Design review of the part shown in the three views and the two pictorial views. Dimensions are in mm from the part's minimum x, y and z. Round coordinates to 2 decimals unless told otherwise and drop trailing zeros. Loops run counter-clockwise (first coordinate to the right, second up) from the corner with the lowest first, then second, coordinate; pieces in that order, holes last. Notation, with made-up numbers: M 77,31 L 97,31 A21 cw 97,45 Z; hole C -30.5,16.5 d1. An arc over 180 degrees is marked long. One line per question, with ' | ' between items. Start each with the question number.
1) For pin 1 Ø2 at (x, z) = (13, 3) entering from +Y, flat-tipped, find the tip position at first contact; note if it passes through.
2) For probe 1 along X at (y, z) = (53, 0.35); probe 2 along X at (y, z) = (55, 1.05); probe 3 along X at (y, z) = (16.5, 2.9), list the stretches that pass through material, from the lowest coordinate up. Write a range as from..to.
3) We need section B-B (y = 58). Give the boundary of the cut face in (x, z), and give its area (3 significant figures).
4) We need section C-C (y = 7). Give the boundary of the cut face in (x, z).
5) We need section A-A (y = 13.5). Give the boundary of the cut face in (x, z), and give its area (3 significant figures).
6) We need section D-D (x = 70.5). Give the boundary of the cut face in (y, z), and give its area (3 significant figures).
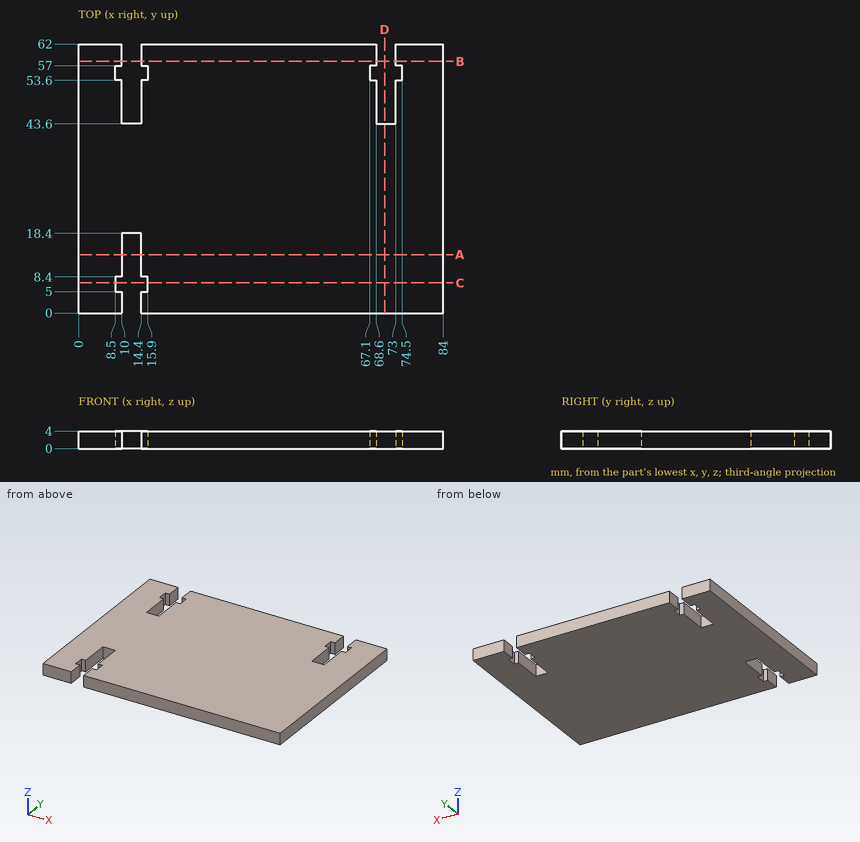
Answers below:
1) pin 1: y = 43.6
2) probe 1: 0..10, 14.4..68.6, 73..84 | probe 2: 0..8.5, 15.9..67.1, 74.5..84 | probe 3: 0..10, 14.4..84
3) outline: M 0,0 L 10,0 L 10,4 L 0,4 Z; M 14.4,0 L 68.6,0 L 68.6,4 L 14.4,4 Z; M 73,0 L 84,0 L 84,4 L 73,4 Z | area: 301 mm^2
4) outline: M 0,0 L 8.5,0 L 8.5,4 L 0,4 Z; M 15.9,0 L 84,0 L 84,4 L 15.9,4 Z
5) outline: M 0,0 L 10,0 L 10,4 L 0,4 Z; M 14.4,0 L 84,0 L 84,4 L 14.4,4 Z | area: 318 mm^2
6) outline: M 0,0 L 43.6,0 L 43.6,4 L 0,4 Z | area: 174 mm^2
